Verification items for this drawing (mm, ordinates from the low corner). Give positions to 0.01 mm unless a question says otherwise; leave off trailing zeros. Order: outer loops, then holes, each group sorted by start corner. A loop starts at its lowest first (then second) coordinate and runs counter-clockwise, first axis right, second up.
(1) Gauge pin test, flat end, axial feed: pin 1 (1 mm diameter, centred on x = 46, y = 1, fed in from -Z). Record the tip position at first contact, or that the pin passes through.
(2) Scan lines: L1, parallel to X at y = 0.7, z = 2.75; L2, parallel to X at y = 1.4, z = 1.5; L3, parallel to Z at x = 82.25, y = 1.2. Record each from-to range of solid material in increasing order.
(3) Sectioned sample at C-C on z = 17.75. Record the cut outline in (x, y).
(4) Sectioned sample at D-D on x = 2.75. Record the cut outline in (y, z).
(5) Sectioned sample at A-A on x = 82.25. Record the cut outline in (y, z), plus the area to 3 significant figures.
(6) Sectioned sample at B-B on y = 1. Count the separate pieces of the cut face and the enclosed holes in it, plus the area to 3 significant figures.
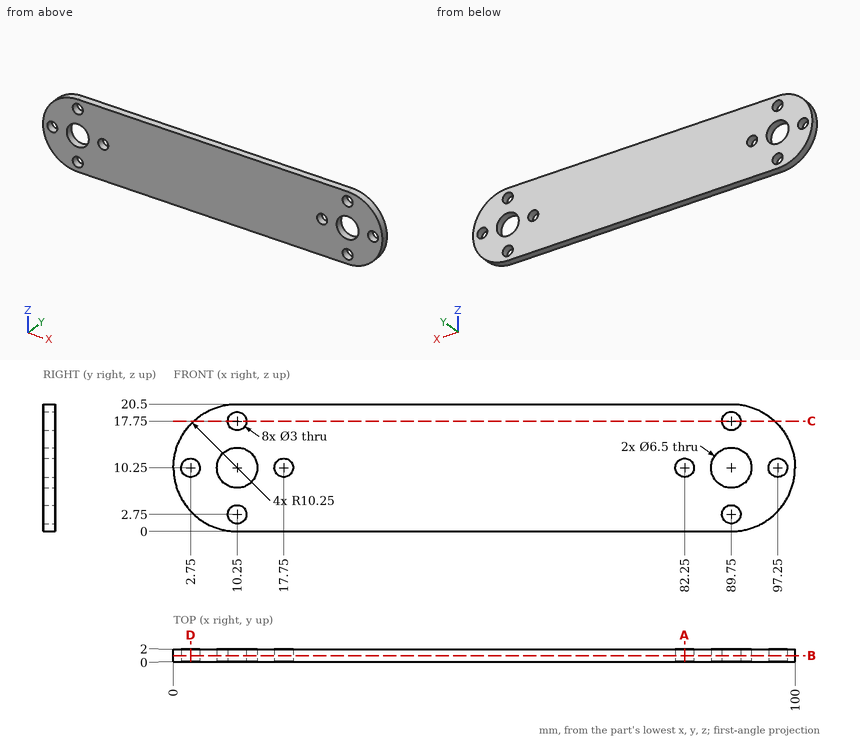
Ans:
1. pin 1: stops at z = 0
2. L1: x = 3.26 to 8.75, 11.75 to 88.25, 91.25 to 96.74
2. L2: x = 4.91 to 9.42, 11.08 to 88.92, 90.58 to 95.09
2. L3: z = 0 to 8.75, 11.75 to 20.5
3. outline: (3.26, 0) - (8.75, 0) - (8.75, 2) - (3.26, 2) - close; (11.75, 0) - (88.25, 0) - (88.25, 2) - (11.75, 2) - close; (91.25, 0) - (96.74, 0) - (96.74, 2) - (91.25, 2) - close
4. outline: (0, 3.26) - (2, 3.26) - (2, 8.75) - (0, 8.75) - close; (0, 11.75) - (2, 11.75) - (2, 17.24) - (0, 17.24) - close
5. outline: (0, 0) - (2, 0) - (2, 8.75) - (0, 8.75) - close; (0, 11.75) - (2, 11.75) - (2, 20.5) - (0, 20.5) - close
5. area: 35.0 mm2
6. separate pieces: 1
6. enclosed holes: 10
6. area: 1,840 mm2
